Autodesk Fusion 360 part; units mm, degrees
sketch "Sketch13" plane through (0, 0, 0) normal (0, 0, 1) x (1, 0, 0)
  line L0 (0, 105) -> (0, 100)
  arc A0 (-16.7, 100.6236) -> (-25, 98.8888) centre (0, 0) ccw
  line L1 (-25, 98.8888) -> (-25, 96.8246)
  arc A1 (-21.35, 97.6943) -> (-25, 96.8246) centre (0, 0) ccw
  line L2 (0, 90) -> (0, 100)
  line L3 (-21.35, 97.6943) -> (-21.35, 90)
  line L4 (0, 90) -> (0, 100)
  line L5 (-16.7, 100.7023) -> (-16.7, 100.6236)
  line L6 (0, 90) -> (-21.35, 90)
  line L7 (0, 105) -> (-12.5, 105)
  line L8 (-16.7, 100.7023) -> (-12.5, 100.7023)
  line L9 (-12.5, 100.7023) -> (-12.5, 105)
  dimension "d41" = 200
  dimension "d42" = 204
  dimension "d54" = 10
  dimension "d66" = 12.5
revolve "Revolve4" add sketch "Sketch13" angle 360 about axis through (0, 105, 0) along (0, -1, 0)
fillet "Fillet2" radius 1 1 edges at (-23.3082, 98.8888, 9.0404)
fillet "Fillet3" radius 1 1 edges at (-19.9052, 90, 7.7205)
sketch "Sketch16" plane through (0, 90, 0) normal (0, -1, 0) x (1, 0, 0)
  circle A0 centre (0, 0) radius 20.35
  circle A1 centre (0, 0) radius 7.75
  circle A2 centre (0, 0) radius 12.5
  dimension "d69" = 15.5
  dimension "d72" = 25
extrude "Extrude7" cut sketch "Sketch16" against normal blind 30 contours A1
extrude "Extrude8" add sketch "Sketch16" along normal blind 50 contours A2
extrude "Extrude9" add sketch "Sketch16" along normal blind 55 and the other way blind -40 contours A1
sketch "Sketch18" plane through (0, 35, 0) normal (0, -1, 0) x (1, 0, 0)
  circle A0 centre (0, 0) radius 7.75
  circle A1 centre (0, 0) radius 2.1
  dimension "d80" = 4.2
extrude "Extrude10" cut sketch "Sketch18" against normal blind 86 contours A1
Read the model definition and answer for the solid it produces. Units are mm, in the model's axes. A direction names the side the tool comes from. Give positions to 0.01 mm unless a question says otherwise; leave off trailing zeros. Order: outer loops, then holes, each group sorted by start corner. A loop starts at its lowest first (then second) coordinate and runs counter-clockwise, first axis right, second up.
(1) For faces 1 (the cylindrical face through (-23.846, 97.457, -7.509)), 2 (the flat face through (-6.1, 100.702, 11.1)), 3 (the flat face through (9, 90, 9)), determine the directions among +Z, -Z, +X, -X, +Y, -Y from which every point of the face is accessible in a straight line to the end or side of a thin tool.
(2) For a pull along Z with two mould halves and no side action, classify faces 4 (the flat face through (0, 105, 8)), 5 (the cylindrical face through (11.923, 65.35, -3.755)), 6 (the cylindrical face through (2.003, 42.395, 0.631)) as released by +Z, released by -Z, zero draft, split by the parting line, or undercut.
(3) Find section B-B (y = 92). Give the vertices of the cut face in (x, z).
(4) Find section A-A (y = 62). Give the vertices of the cut face in (x, z).
(5) Straight lines are drawn through the part: L1, parallel to Z at x = 0, y = 39; L2, parallel to Z at x = 0, y = 63; L3, parallel to Y at x = 9.5, z = 13. For each, find the intervals that lie inside material, in ascending order.
(6) Given pin 1 (12 mm diameter, centred on y = 77.5, z = 9.5, fed in from +X); pin 2 (1.5 mm diameter, centred on y = 60.5, z = -3.5, fed in from +X); pin 3 (12.5 mm diameter, centred on x = 0, z = 0, fed in from -Y); pin 4 (5 mm diameter, centred on x = 0, z = 0, fed in from +Y), each flat-ended and moving along its own axis, determine where each tip first touches the part or whether it passes through.
Result sheet:
1. face 1: +Y, -Y
1. face 2: +Y
1. face 3: -Y
2. face 4: zero draft
2. face 5: split by the parting line
2. face 6: undercut
3. outline: circle Ø42.7 at (0, 0); hole circle Ø15.5 at (0, 0)
4. outline: circle Ø25 at (0, 0); hole circle Ø15.5 at (0, 0)
5. L1: z = -7.75 to -2.1, 2.1 to 7.75
5. L2: z = -12.5 to -7.75, 7.75 to 12.5
5. L3: y = 90 to 100.7
6. pin 1: stops at x = 12
6. pin 2: stops at x = 12.19
6. pin 3: stops at y = 35
6. pin 4: stops at y = 50
